The drawing under review shows one solid part. Ordinate dimensions are in mm from its lowest x, y, z. A direction names the side the tool comes from. Round coordinates to 2 decimals unless told otherwise and drop trailing zeros. Order: outer loops, then holes, each group sorted by start corner. A loop starts at its lowest first (then second) coordinate and runs counter-clockwise, first axis right, second up. Notation, with made-up numbers: M 79,79.25 L 112,79.25 A10 ccw 112,86.25 Z; hole C 17,79.25 d8. An arc over 180 degrees is marked long. Answer as a JSON object with one key per item and string values. Group by question number.
1. To check wall thickness, follow probe 1 along X at (y, z) = (0.75, 2.55); probe 2 along Y at (x, z) = (1, 2.85); probe 3 along Y at (x, z) = (2.6, 2). State the ranges of each line that lie inside material, in increasing order. Write a range as [from, to].
2. Add section C-C on z = 2.5. State the section outline as (x, y) points, and give its area (3 significant figures).
3. Add section A-A on x = 2.5. State the section outline as (y, z) points.
4. Machinability: for the marked faces 4, 5 and 6, which of the approach directions +Z, -Z, +X, -X, +Y, -Y give a long, thin tool a straight path to every point of the face, cutting with its end or side? Answer none if there is none.
5. Clearance check with flat-ended pins moving along their axes: P1, Ø0.8, axis at y = 0.5, z = 4, coming from the +X side (3 decimals); P2, Ø0.8, axis at x = 4, y = 0.5, coming from the +Z side (3 decimals); P3, Ø1, axis at x = 2.5, y = 6, coming from the +Z side. State where each tip first meets the part, or that it passes through.
6. Add section D-D on y = 4. State the section outline as (x, z) points, and give its area (3 significant figures).
7. Add section B-B on y = 0.5. State the section outline as (x, z) points, and give its area (3 significant figures).
8. Mouldability with a two-part tool opening along Z and no side actions: class the marked faces 1, 2 and 3 as released by +Z, released by -Z, zero draft, split by the parting line, or undercut.
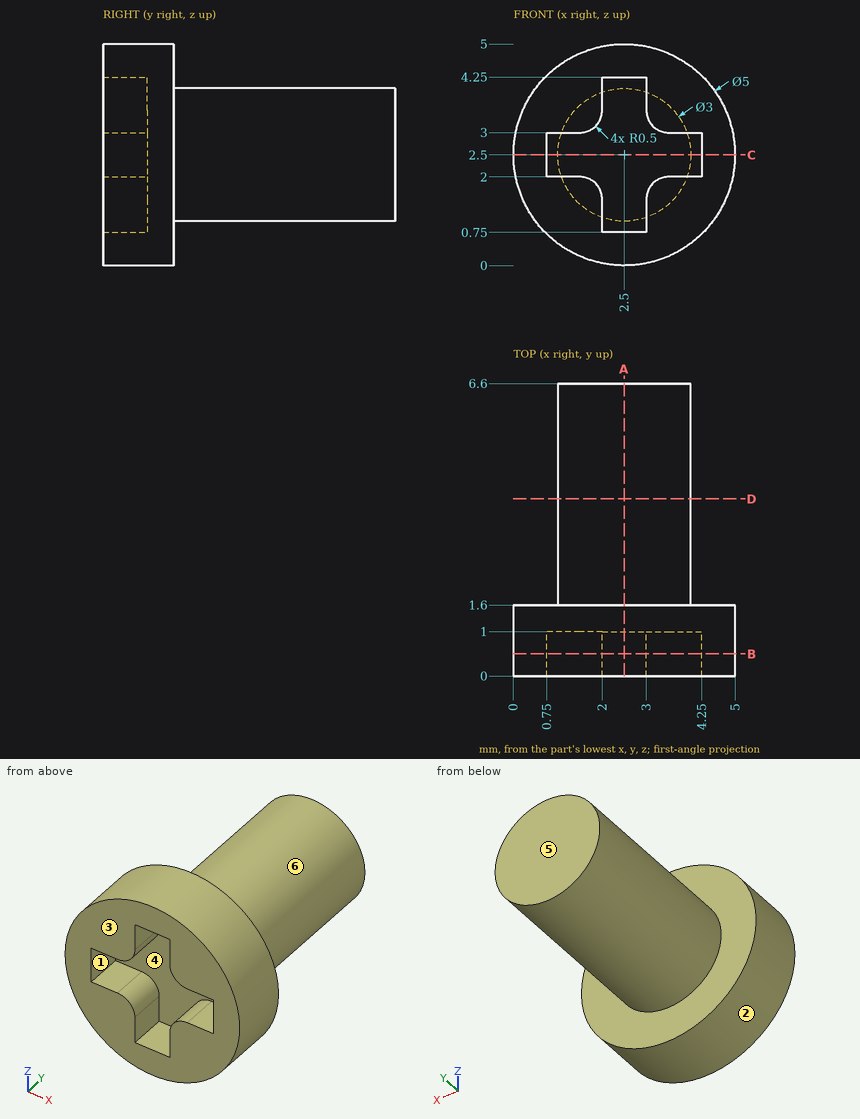
Recorded:
{
 "1": {"probe 1": "x = [0, 0.75], [4.25, 5]", "probe 2": "y = [1, 1.6]", "probe 3": "y = [1, 6.6]"},
 "2": {"outline": "M 0,0 L 0.75,0 L 0.75,1 L 4.25,1 L 4.25,0 L 5,0 L 5,1.6 L 4,1.6 L 4,6.6 L 1,6.6 L 1,1.6 L 0,1.6 Z", "area": "19.5 mm²"},
 "3": {"outline": "M 0,0 L 1.6,0 L 1.6,1 L 6.6,1 L 6.6,4 L 1.6,4 L 1.6,5 L 0,5 L 0,4.25 L 1,4.25 L 1,0.75 L 0,0.75 Z"},
 "4": {"face 4": "-Y", "face 5": "+Z, -Z, +X, -X, +Y", "face 6": "+Y"},
 "5": {"P1": "stops at x = 4.745", "P2": "stops at z = 4.745", "P3": "stops at z = 4"},
 "6": {"outline": "C 2.5,2.5 d3", "area": "7.07 mm²"},
 "7": {"outline": "C 2.5,2.5 d5; hole M 0.75,2 L 1.5,2 A0.5 cw 2,1.5 L 2,0.75 L 3,0.75 L 3,1.5 A0.5 cw 3.5,2 L 4.25,2 L 4.25,3 L 3.5,3 A0.5 cw 3,3.5 L 3,4.25 L 2,4.25 L 2,3.5 A0.5 cw 1.5,3 L 0.75,3 Z", "area": "13.4 mm²"},
 "8": {"face 1": "undercut", "face 2": "split by the parting line", "face 3": "zero draft"}
}
